Check sheet for the modelled part. Datum: model origin and axes. Units: mm. A direction names the side the tool comes from. Round coordinates to 2 decimals unless told otherwise and drop trailing zeros. Write each loop counter-clockwise with the first axis right and the second up, starting at its lowest first coordinate (ties: lowest second). Pieces come first, ordered by that corner, then holes. Notation, with made-up numbers: M 51.25,59 L 68.25,59 A26 ccw 68.25,78 Z; hole C 43.25,17.5 d4. An arc over 180 degrees is marked long. Put each result on its own line as item: value.
```python
from build123d import *

# Parameters (mm, degrees)
SKETCH2_R           = 8
BOSS_EXTRUDE1_DEPTH = 40
CUT_EXTRUDE1_DEPTH  = 40
SKETCH4_R           = 4.5
BOSS_EXTRUDE2_DEPTH = 32


with BuildPart() as part:
    # Sketch2 → Boss-Extrude1 (new body)
    with BuildSketch(Plane.XY):
        with BuildLine():
            Line((0, 0), (36, 0))
            Line((36, 0), (36, 32))
            Line((36, 32), (0, 32))
            ThreePointArc((0, 32), (-16, 16), (0, 0))
        make_face()
        with Locations((0, 16)):
            Circle(SKETCH2_R, mode=Mode.SUBTRACT)
    extrude(amount=BOSS_EXTRUDE1_DEPTH)

    # Sketch3 → Cut-Extrude1 (cut)
    with BuildSketch(Plane(origin=(0, 32, 0), x_dir=(1, 0, 0), z_dir=(0, 1, 0))):
        Polygon((26, -11), (0, -11), (0, -29), (25.876198368, -29), align=None)
        Polygon((0, -11), (-16, -11), (-16.123801632, -29), (0, -29), align=None)
    extrude(amount=-CUT_EXTRUDE1_DEPTH, mode=Mode.SUBTRACT)

    # Sketch4 → Boss-Extrude2 (add)
    with BuildSketch(Plane(origin=(36, 0, 0), x_dir=(0, 0, -1), z_dir=(1, 0, 0))):
        with Locations((-20, 16)):
            Circle(SKETCH4_R)
    extrude(amount=BOSS_EXTRUDE2_DEPTH)


solid = part.part
```
1. Cross-section at A-A (x = 19.5). Enter the section's corners in (y, z), then the cut area to 3 significant figures.
Computed values:
outline: M 0,0 L 32,0 L 32,11 L 0,11 Z; M 0,29 L 32,29 L 32,40 L 0,40 Z
area: 704 mm2
2. Access from +Z, -Z, +X, -X, +Y, -Y to the whole of each face (thin tool, end or side, straight path). Record for faces 1 (the flat face through (10, 16, 11)), 2 (the cylindrical face through (51.78, 19.04, 23.32)), 3 (the flat face through (68, 16, 20)).
Computed values:
face 1: -X, +Y, -Y
face 2: +X
face 3: +Z, -Z, +X, +Y, -Y
3. Depth check by flat-ended pin: pin 1 Ø12 at (y, z) = (8, 25) entering from -X; pin 2 Ø5 at (y, z) = (14, 27) entering from -X; pin 3 Ø5 at (x, z) = (-7.5, 10.5) entering from -Y. Enter the tip coordinate at first touch or a pass-through.
Computed values:
pin 1: stops at x = -15.61
pin 2: stops at x = -15.99
pin 3: stops at y = 0.8
4. Cross-section at B-B (y = 16). Enter the section's corners in (x, z), then the cut area to 3 significant figures.
Computed values:
outline: M -16,0 L -8,0 L -8,11 L -16,11 Z; M -16,29 L -8,29 L -8,40 L -16,40 Z; M 8,0 L 36,0 L 36,15.5 L 68,15.5 L 68,24.5 L 36,24.5 L 36,40 L 8,40 L 8,29 L 25.88,29 L 26,11 L 8,11 Z
area: 1,260 mm2
5. Cross-section at D-D (z = 17). Enter the section's corners in (x, y), then the cut area to 3 significant figures.
Computed values:
outline: M 25.96,0 L 36,0 L 36,12.65 L 68,12.65 L 68,19.35 L 36,19.35 L 36,32 L 25.96,32 Z
area: 536 mm2
6. Release check for a two-part mould opening along X. For faces 4 (the flat face through (9, 16, 29)), 5 (the cylindrical face through (-1.73, 8.19, 34.42)), 6 (the flat face through (36, 16, 15)) record: +X half, -X half, draft (parallel to the pull), parting line (faces both ways), or undercut.
Computed values:
face 4: draft
face 5: undercut
face 6: +X half
7. Scan lines: probe 1 along Y at (x, z) = (0, 7); probe 2 along X at (y, z) = (16, 3.5); probe 3 along Z at (x, y) = (15, 17.5). Record each from-to range of solid material in increasing order.
Computed values:
probe 1: y = 0 to 8, 24 to 32
probe 2: x = -16 to -8, 8 to 36
probe 3: z = 0 to 11, 29 to 40
8. Cross-section at C-C (z = 34). Enter the section's corners in (x, y).
Computed values:
outline: M 0,0 L 36,0 L 36,32 L 0,32 A16 ccw Z; hole C 0,16 d16
